Model file for the job. Use its own axes, mm. Face numbers are marked on the shaded views. A direction names the side the tool comes from. Give positions to 0.01 mm unless a question says otherwise; leave off trailing zeros. Loops run counter-clockwise (first coordinate to the right, second up) from the corner with the lowest first, then second, coordinate; pieces in that order, holes last. Notation, with made-up numbers: M 17.5,6.25 L 51.5,6.25 A34 ccw 51.5,45.25 Z; hole C -24,-18.5 d11. An arc over 180 degrees is marked long. Answer in a Markdown table with one row per item.
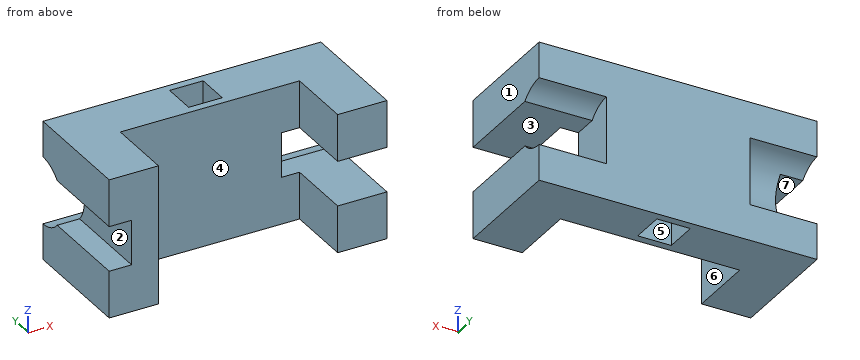
```python
from build123d import *

# Parameters (mm, degrees)
SKETCH1_W           = 15
SKETCH1_H           = 15
BOSS_EXTRUDE2_DEPTH = 62
SKETCH2_W           = 20
SKETCH2_H           = 52
CUT_EXTRUDE1_DEPTH  = 10
CUT_EXTRUDE2_DEPTH  = 30
SKETCH5_W           = 20
SKETCH5_H           = 52
CUT_EXTRUDE4_DEPTH  = 30
CUT_EXTRUDE5_START  = -30
CUT_EXTRUDE5_DEPTH  = 30


with BuildPart() as part:
    # Sketch1 → Boss-Extrude2 (new body)
    with BuildSketch(Plane.XY):
        Polygon((0, 0), (0, 52), (124, 52), (124, 0.029795627), (102, 0.029795627), (102, 30), (22, 30), (22, 0), align=None)
        with Locations((62, 41)):
            Rectangle(SKETCH1_W, SKETCH1_H, mode=Mode.SUBTRACT)
    extrude(amount=BOSS_EXTRUDE2_DEPTH)

    # Sketch2 → Cut-Extrude1 (cut)
    with BuildSketch(Plane.ZY):
        with Locations((31, 26)):
            Rectangle(SKETCH2_W, SKETCH2_H)
    extrude(amount=-CUT_EXTRUDE1_DEPTH, mode=Mode.SUBTRACT)

    # Sketch3 → Cut-Extrude2 (cut)
    with BuildSketch(Plane.ZY):
        with BuildLine():
            Line((16, 52), (46, 52))
            ThreePointArc((46, 52), (31, 37), (16, 52))
        make_face()
    extrude(amount=-CUT_EXTRUDE2_DEPTH, mode=Mode.SUBTRACT)

    # Sketch5 → Cut-Extrude4 (cut)
    with BuildSketch(Plane(origin=(124, 0, 0), x_dir=(0, 0, -1), z_dir=(1, 0, 0))):
        with Locations((-31, 26)):
            Rectangle(SKETCH5_W, SKETCH5_H)
    extrude(amount=-CUT_EXTRUDE4_DEPTH, mode=Mode.SUBTRACT)

    # Sketch6 → Cut-Extrude5 (cut)
    with BuildSketch(Plane(origin=(124, 0, 0), x_dir=(0, 0, -1), z_dir=(1, 0, 0)).offset(CUT_EXTRUDE5_START)):
        with BuildLine():
            Line((-46, 52), (-16, 52))
            ThreePointArc((-16, 52), (-31, 37), (-46, 52))
        make_face()
    extrude(amount=CUT_EXTRUDE5_DEPTH, mode=Mode.SUBTRACT)


solid = part.part
```
Q1. Probe probe 1 along X at (y, z) = (13.5, 46); probe 2 along Y at (x, z) = (64, 31); probe 3 along Z at (x, y) = (118, 16). List the from-to ranges inside material, lowest first.
Reported:
| item | result |
|---|---|
| probe 1 | 0 to 22, 102 to 124 |
| probe 2 | 30 to 33.5, 48.5 to 52 |
| probe 3 | 0 to 21, 41 to 62 |
Q2. Saw through at D-D (x = 44.5). Give the cut face in (y, z), and give its area (3 significant figures).
Reported:
| item | result |
|---|---|
| outline | M 30,0 L 52,0 L 52,62 L 30,62 Z |
| area | 1,360 mm² |
Q3. Saw through at B-B (z = 11). Give the cut face in (x, y).
Reported:
| item | result |
|---|---|
| outline | M 0,0 L 22,0 L 22,30 L 102,30 L 102,0.03 L 124,0.03 L 124,52 L 0,52 Z; hole M 54.5,33.5 L 69.5,33.5 L 69.5,48.5 L 54.5,48.5 Z |
Q4. Saw through at C-C (z = 31). Give the cut face in (x, y), and give its area (3 significant figures).
Reported:
| item | result |
|---|---|
| outline | M 10,0 L 22,0 L 22,30 L 94,30 L 94,52 L 30,52 L 30,37 L 10,37 Z; hole M 54.5,33.5 L 69.5,33.5 L 69.5,48.5 L 54.5,48.5 Z |
| area | 1,680 mm² |
Q5. Saw through at A-A (x = 104.5). Give the cut face in (y, z), and give its area (3 significant figures).
Reported:
| item | result |
|---|---|
| outline | M 0.03,0 L 52,0 L 52,16 A15 cw 40.82,21 L 0.03,21 Z; M 0.03,41 L 40.82,41 A15 cw 52,46 L 52,62 L 0.03,62 Z |
| area | 2,110 mm² |
Q6. 3-axis set-ups, long thin cutter, end or side, ignore diameter. For the marked faces 5, 6 and 7: which of +Z, -Z, +X, -X, +Y, -Y reach the whole face in a straight line?
Reported:
| item | result |
|---|---|
| face 5 | +Z, -Z |
| face 6 | +Z, -Z, -Y |
| face 7 | -X, +Y, -Y |
Q7. Drop flat-ended pins along their axis: pin 1 (2 mm diameter, centred on x = 107.5, z = 14.5, fed in from -Y); pin 2 (12 mm diameter, centred on y = 44.5, z = 33, fed in from -X); pin 3 (16.5 mm diameter, centred on y = 42, z = 35.5, fed in from -X); pin 4 (4 mm diameter, centred on x = 60, z = 37, fed in from -Y). Give the stop position or say it passes through.
Reported:
| item | result |
|---|---|
| pin 1 | y = 0.03 |
| pin 2 | x = 30 |
| pin 3 | x = 0 |
| pin 4 | y = 30 |
Q8. Mould opens along X. For the marked faces 1, 2, 3 and 4 say: released by +X, released by -X, zero draft, split by the parting line, or undercut.
Reported:
| item | result |
|---|---|
| face 1 | released by +X |
| face 2 | released by -X |
| face 3 | zero draft |
| face 4 | undercut |
